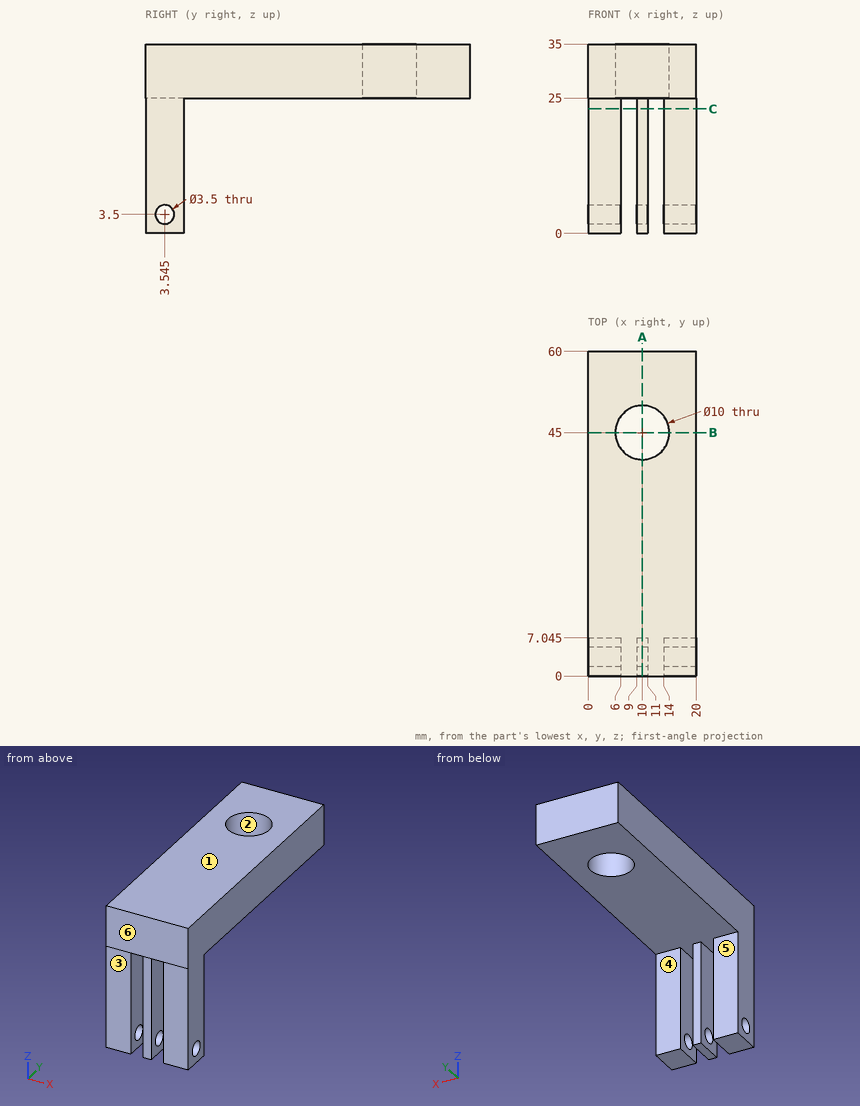
Job drawing, mm, ordinate dimensions from the low corner. One solid piece. A direction names the side the tool comes from. Coordinates: 2 decimals unless noted, no trailing zeros. Write each loop counter-clockwise with the first axis right and the second up, starting at its lowest first coordinate (ties: lowest second). Pieces come first, ordered by that corner, then holes.
Item 1: Probe line 1 (Y direction, x = 10.25, z = 26); line 2 (Z direction, x = 15.25, y = 52); line 3 (Y direction, x = 16, z = 18) (1 decimal). List the from-to ranges inside material, lowest first.
Item 2: Slice it at A-A (x = 10). Count the separate pieces of the cut face and the enclosed holes in it.
Item 3: Mould opens along Y. For the marked faces 1, 2, 3 and 4 say: released by +Y, released by -Y, zero draft, split by the parting line, or undercut.
Item 4: Slice it at C-C (z = 23). Write the cut outline in (x, y) (1 decimal).
Item 5: Which spindle directions (+Z, -Z, +X, -X, +Y, -Y) get a long thin tool onto all of the face, cutting with end or side? Do the marked faces 5 and 6. Say none if no direction does.
Item 6: Slice it at B-B (y = 45). Write the cut outline in (x, z), and give its area (3 significant figures).
Item 7: Pin check, flat tips, straight feed: pin 1 (6 mm diameter, centred on x = 10, y = 45, fed in from +Z); pin 2 (8 mm diameter, centred on x = 11, y = 36.5, fed in from -Z); pin 3 (6 mm diameter, centred on x = 16.5, z = 13.5, fed in from +Y) (1 decimal). Stop position of each tip, or through.
Results found:
1. line 1: y = 0 to 40.01, 49.99 to 60
1. line 2: z = 25 to 35
1. line 3: y = 0 to 7
2. separate pieces: 2
2. enclosed holes: 1
3. face 1: zero draft
3. face 2: undercut
3. face 3: released by -Y
3. face 4: released by +Y
4. outline: (0, 0) - (6, 0) - (6, 7) - (0, 7) - close; (9, 0) - (11, 0) - (11, 7) - (9, 7) - close; (14, 0) - (20, 0) - (20, 7) - (14, 7) - close
5. face 5: -Z, +X, -X, +Y
5. face 6: +Z, -Z, +X, -X, -Y
6. outline: (0, 25) - (5, 25) - (5, 35) - (0, 35) - close; (15, 25) - (20, 25) - (20, 35) - (15, 35) - close
6. area: 100 mm2
7. pin 1: passes through
7. pin 2: stops at z = 25
7. pin 3: stops at y = 7
